CAD build for the part. Positions are in the model's coordinates, mm. Face numbers are marked on the shaded views. A direction names the side the tool comes from. Give positions to 0.01 mm unless a question says otherwise; leave off trailing zeros. Write each loop counter-clockwise with the first axis right and the second up, starting at its lowest first coordinate (ties: lowest second). Pieces come first, ordered by that corner, then holes. Notation, with made-up numbers: (40, 35) -> (46, 35) arc R31 cw to (46, 68) -> close; hole circle Ø8 at (-32, 3.5). An arc over 180 degrees is marked (long way). Use one line per item in the form item = value. Start each with the question number.
from build123d import *

# Parameters (mm, degrees)
SKETCH1_R           = 38.1
BOSS_EXTRUDE1_DEPTH = 20.1
SKETCH4_R           = 3.125
CUT_EXTRUDE3_DEPTH  = 134.421728778
SKETCH6_R           = 3.125
CUT_EXTRUDE4_DEPTH  = 134.889662183
SKETCH7_R           = 3.125
CUT_EXTRUDE5_DEPTH  = 154.333276804


with BuildPart() as part:
    # Sketch1 → Boss-Extrude1 (new body)
    with BuildSketch(Plane.XY):
        with BuildLine():
            Line((-87.199197341, 83.680917653), (-92.083580619, 80.860917653))
            ThreePointArc((-92.083580619, 80.860917653), (-92.549506445, 80.253711294), (-92.449606022, 79.494892249))
            Line((-92.449606022, 79.494892249), (-83.449606022, 63.906434981))
            ThreePointArc((-83.449606022, 63.906434981), (-83.3497056, 63.147615936), (-83.815631426, 62.540409577))
            Line((-83.815631426, 62.540409577), (-97.240798671, 54.789385655))
            ThreePointArc((-97.240798671, 54.789385655), (-97.999617716, 54.689485232), (-98.606824075, 55.155411058))
            Line((-98.606824075, 55.155411058), (-107.606824075, 70.743868326))
            ThreePointArc((-107.606824075, 70.743868326), (-108.214030434, 71.209794153), (-108.972849479, 71.10989373))
            Line((-108.972849479, 71.10989373), (-113.857232756, 68.28989373))
            ThreePointArc((-113.857232756, 68.28989373), (-114.221904453, 67.692926638), (-114.106124766, 67.003035183))
            Line((-114.106124766, 67.003035183), (-96.816210848, 37.056025818))
            ThreePointArc((-96.816210848, 37.056025818), (-95.976342212, 33.509634544), (-97.224589096, 30.085579914))
            ThreePointArc((-97.224589096, 30.085579914), (-107.297524567, -0.277987315), (-97.224589096, -30.641554544))
            ThreePointArc((-97.224589096, -30.641554544), (-95.976342212, -34.065609174), (-96.816210848, -37.612000448))
            Line((-96.816210848, -37.612000448), (-114.106124766, -67.559009813))
            ThreePointArc((-114.106124766, -67.559009813), (-114.221904453, -68.248901268), (-113.857232756, -68.84586836))
            Line((-113.857232756, -68.84586836), (-108.972849479, -71.66586836))
            ThreePointArc((-108.972849479, -71.66586836), (-108.214030434, -71.765768783), (-107.606824075, -71.299842956))
            Line((-107.606824075, -71.299842956), (-98.606824075, -55.711385688))
            ThreePointArc((-98.606824075, -55.711385688), (-97.999617716, -55.245459862), (-97.240798671, -55.345360285))
            Line((-97.240798671, -55.345360285), (-83.815631426, -63.096384207))
            ThreePointArc((-83.815631426, -63.096384207), (-83.3497056, -63.703590566), (-83.449606022, -64.462409611))
            Line((-83.449606022, -64.462409611), (-92.449606022, -80.050866879))
            ThreePointArc((-92.449606022, -80.050866879), (-92.549506445, -80.809685924), (-92.083580619, -81.416892283))
            Line((-92.083580619, -81.416892283), (-87.199197341, -84.236892283))
            ThreePointArc((-87.199197341, -84.236892283), (-86.499872826, -84.25422369), (-85.960299143, -83.809009813))
            Line((-85.960299143, -83.809009813), (-68.670385225, -53.862000448))
            ThreePointArc((-68.670385225, -53.862000448), (-66.019054608, -51.361457236), (-62.429612873, -50.730443433))
            ThreePointArc((-62.429612873, -50.730443433), (-31.097524567, -44.272077827), (-9.838371733, -20.366876204))
            ThreePointArc((-9.838371733, -20.366876204), (-7.497176881, -17.573835377), (-4.005977629, -16.527987315))
            Line((-4.005977629, -16.527987315), (30.573850208, -16.527987315))
            ThreePointArc((30.573850208, -16.527987315), (31.229203577, -16.283309737), (31.563856396, -15.669011238))
            Line((31.563856396, -15.669011238), (31.563856396, -10.029011238))
            ThreePointArc((31.563856396, -10.029011238), (31.270963178, -9.321904457), (30.563856396, -9.029011238))
            Line((30.563856396, -9.029011238), (12.563856396, -9.029011238))
            ThreePointArc((12.563856396, -9.029011238), (11.856749615, -8.736118019), (11.563856396, -8.029011238))
            Line((11.563856396, -8.029011238), (11.563856396, 7.473036608))
            ThreePointArc((11.563856396, 7.473036608), (11.856749615, 8.180143389), (12.563856396, 8.473036608))
            Line((12.563856396, 8.473036608), (30.563856396, 8.473036608))
            ThreePointArc((30.563856396, 8.473036608), (31.270963178, 8.765929827), (31.563856396, 9.473036608))
            Line((31.563856396, 9.473036608), (31.563856396, 15.113036608))
            ThreePointArc((31.563856396, 15.113036608), (31.229203577, 15.727335107), (30.573850208, 15.972012685))
            Line((30.573850208, 15.972012685), (-4.005977629, 15.972012685))
            ThreePointArc((-4.005977629, 15.972012685), (-7.497176881, 17.017860747), (-9.838371733, 19.810901574))
            ThreePointArc((-9.838371733, 19.810901574), (-31.097524567, 43.716103197), (-62.429612873, 50.174468803))
            ThreePointArc((-62.429612873, 50.174468803), (-66.019054608, 50.805482606), (-68.670385225, 53.306025818))
            Line((-68.670385225, 53.306025818), (-85.960299143, 83.253035183))
            ThreePointArc((-85.960299143, 83.253035183), (-86.499872826, 83.69824906), (-87.199197341, 83.680917653))
        make_face()
        with BuildLine():
            ThreePointArc((-91.68717238, -52.778245227), (-93.492634957, -50.425320587), (-93.105520819, -47.484896787))
            Line((-93.105520819, -47.484896787), (-87.30204773, -37.432986536))
            ThreePointArc((-87.30204773, -37.432986536), (-84.94912309, -35.627523959), (-82.00869929, -36.014638096))
            Line((-82.00869929, -36.014638096), (-74.690784628, -40.239638096))
            ThreePointArc((-74.690784628, -40.239638096), (-72.885322051, -42.592562736), (-73.272436189, -45.532986536))
            Line((-73.272436189, -45.532986536), (-79.075909278, -55.584896787))
            ThreePointArc((-79.075909278, -55.584896787), (-81.428833918, -57.390359364), (-84.369257718, -57.003245227))
            Line((-84.369257718, -57.003245227), (-91.68717238, -52.778245227))
        make_face(mode=Mode.SUBTRACT)
        with Locations((-56.497524567, -0.277987315)):
            Circle(SKETCH1_R, mode=Mode.SUBTRACT)
        with BuildLine():
            Line((-74.690784628, 39.683663466), (-82.00869929, 35.458663466))
            ThreePointArc((-82.00869929, 35.458663466), (-84.94912309, 35.071549329), (-87.30204773, 36.877011906))
            Line((-87.30204773, 36.877011906), (-93.105520819, 46.928922157))
            ThreePointArc((-93.105520819, 46.928922157), (-93.492634957, 49.869345957), (-91.68717238, 52.222270597))
            Line((-91.68717238, 52.222270597), (-84.369257718, 56.447270597))
            ThreePointArc((-84.369257718, 56.447270597), (-81.428833918, 56.834384734), (-79.075909278, 55.028922157))
            Line((-79.075909278, 55.028922157), (-73.272436189, 44.977011906))
            ThreePointArc((-73.272436189, 44.977011906), (-72.885322051, 42.036588106), (-74.690784628, 39.683663466))
        make_face(mode=Mode.SUBTRACT)
        with BuildLine():
            ThreePointArc((6.563856396, -4.502987315), (5.428895173, -7.243026092), (2.688856396, -8.377987315))
            Line((2.688856396, -8.377987315), (-8.918089783, -8.377987315))
            ThreePointArc((-8.918089783, -8.377987315), (-11.65812856, -7.243026092), (-12.793089783, -4.502987315))
            Line((-12.793089783, -4.502987315), (-12.793089783, 3.947012685))
            ThreePointArc((-12.793089783, 3.947012685), (-11.65812856, 6.687051462), (-8.918089783, 7.822012685))
            Line((-8.918089783, 7.822012685), (2.688856396, 7.822012685))
            ThreePointArc((2.688856396, 7.822012685), (5.428895173, 6.687051462), (6.563856396, 3.947012685))
            Line((6.563856396, 3.947012685), (6.563856396, -4.502987315))
        make_face(mode=Mode.SUBTRACT)
    extrude(amount=BOSS_EXTRUDE1_DEPTH)

    # Sketch4 → Cut-Extrude3 (cut, through all)
    with BuildSketch(Plane(origin=(-28.420602652, -16.408642592, 0), x_dir=(0, 0, -1), z_dir=(0.8660254037844387, 0.49999999999999983, 0))):
        with Locations(Location((-10.05, 106.679392982, 0), (0, 0, 90))):
            Circle(SKETCH4_R)
    extrude(amount=-CUT_EXTRUDE3_DEPTH, mode=Mode.SUBTRACT)

    # Sketch6 → Cut-Extrude4 (cut, through all)
    with BuildSketch(Plane(origin=(-28.179858575, 16.269648934, 0), x_dir=(0, 0, -1), z_dir=(0.8660254037844342, -0.5000000000000079, 0))):
        with Locations(Location((-10.05, -107.160881135, 0), (0, 0, 90))):
            Circle(SKETCH6_R)
    extrude(amount=-CUT_EXTRUDE4_DEPTH, mode=Mode.SUBTRACT)

    # Sketch7 → Cut-Extrude5 (cut, through all)
    with BuildSketch(Plane(origin=(0, 15.972012685, 0), x_dir=(1, 0, 0), z_dir=(0, 1, 0))):
        with Locations(Location((22.173850208, -10.05, 0), (0, 0, 180))):
            Circle(SKETCH7_R)
    extrude(amount=-CUT_EXTRUDE5_DEPTH, mode=Mode.SUBTRACT)


solid = part.part
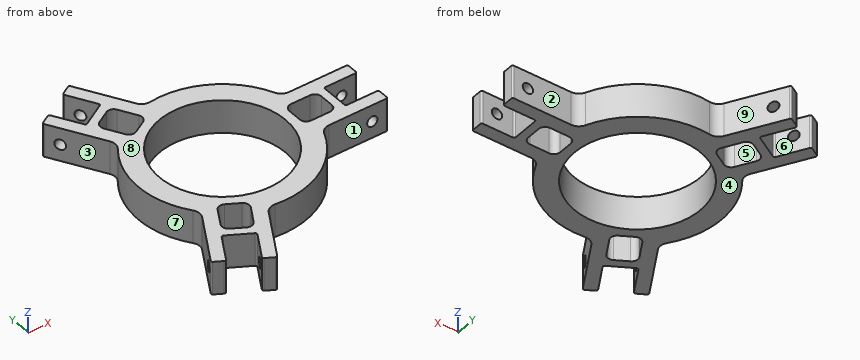
1) Two-plate mould, pull along X, no slides. Class the marked faces 6, 7, 8 and 9: released by +X, released by -X, zero draft, split by the parting line, or undercut.
2) Cut at C-C (x = -40). Give the cut face in (y, z), and give its area (3 significant figures).
3) Wall check: line 1 along Y through (x, z) = (24.5, 17.25); line 2 along Y through (x, z) = (-78, 8); line 3 along X through (y, z) = (-10, 12). Give the ranges that are in metal, low to high. Write a range as from..to.
4) 3-axis set-ups, long thin cutter, end or side, ignore diameter. For the marked faces 1, 2, 3, 4 and 5: which of +Z, -Z, +X, -X, +Y, -Y reach the whole face in a straight line?
5) Cut at B-B (z = 10.05). State how many separate pieces and enclosed holes the cut face has, and give its area (3 significant figures).
6) Cut at A-A (x = -70.5). Give the cut face in (y, z).
7) Pin check, flat tips, straight feed: pin 1 (1.5 mm diameter, centred on y = -57, z = 5.5, fed in from -X); pin 2 (1 mm diameter, centred on y = -29.5, z = 7, fed in from -X); pin 3 (3 mm diameter, centred on y = -40, z = 6.5, fed in from +X). Stop position of each tip, or through.
Final values:
q1.face_6 = undercut
q1.face_7 = released by -X
q1.face_8 = zero draft
q1.face_9 = released by +X
q2.outline = (-48.32, 0) -> (-34.62, 0) -> (-34.62, 20.1) -> (-48.32, 20.1) -> close; (34.07, 0) -> (47.77, 0) -> (47.77, 20.1) -> (34.07, 20.1) -> close
q2.area = 551 mm^2
q3.line_1 = -16.53..-9.03, 8.47..15.97
q3.line_2 = -70.02..-53.72, -38.33..-31.73, 31.17..37.77, 53.17..69.47
q3.line_3 = -106.36..-93.34, -19.66..19.73, 24.62..31.56
q4.face_1 = +Z, -Z, +X, -Y
q4.face_2 = +Z, -Z, +X, +Y
q4.face_3 = +Z, -Z, -X
q4.face_4 = -Z, +X, -X, +Y, -Y
q4.face_5 = +Z, -Z
q5.separate_pieces = 7
q5.enclosed_holes = 4
q5.area = 5,050 mm^2
q6.outline = (-57.03, 0) -> (-35.71, 0) -> (-35.71, 20.1) -> (-57.03, 20.1) -> close; (35.16, 0) -> (56.48, 0) -> (56.48, 20.1) -> (35.16, 20.1) -> close
q7.pin_1 = -108.44
q7.pin_2 = -98.4
q7.pin_3 = -23.04
